CAD build for the part. Positions are in the model's coordinates, mm. Face numbers are marked on the shaded views. Coordinates: 2 decimals unless noted, no trailing zeros. Write each loop counter-clockwise with the first axis right and the second up, starting at its lowest first coordinate (ties: lowest second). Pieces come first, ordered by that corner, then holes.
```python
from build123d import *

# Parameters (mm, degrees)
F0_R          = 8.875
F1_DEPTH      = 5
F1_DEPTH_BACK = 5
F2_DEPTH      = 4
F2_DEPTH_BACK = 4
F3_SIZE       = 1


# Not quite as in the source:
# - a feature names something its author has since deleted; it is built from what else it names


with BuildPart() as f1:
    # F0 (on Front) → F1 (new body, two sides)
    with BuildSketch(Plane.XZ) as f1_sk:
        with BuildLine():
            ThreePointArc((-5, 9.0906889178), (-5.2804178338, -8.9307229551), (10.375, 0))
            ThreePointArc((10.375, 0), (8.9307229551, 5.2804178338), (5, 9.0906889178))
            Line((5, 9.0906889178), (5, 8.9453239366))
            Line((5, 8.9453239366), (-5, 8.9453239366))
            Line((-5, 8.9453239366), (-5, 9.0906889178))
        make_face()
        Circle(F0_R, mode=Mode.SUBTRACT)
        with BuildLine():
            Line((5, 8.9453239366), (5, 9.0906889178))
            ThreePointArc((5, 9.0906889178), (0, 10.375), (-5, 9.0906889178))
            Line((-5, 9.0906889178), (-5, 8.9453239366))
            Line((-5, 8.9453239366), (5, 8.9453239366))
        make_face()
    extrude(amount=F1_DEPTH)
    extrude(f1_sk.sketch, amount=-F1_DEPTH_BACK)

    # F0 (on Front) → F2 (join, two sides)
    with BuildSketch(Plane.XZ) as f2_sk:
        with BuildLine():
            ThreePointArc((-5, 9.0906889178), (0, 10.375), (5, 9.0906889178))
            Line((5, 9.0906889178), (5, 13.9453239366))
            Line((5, 13.9453239366), (-5, 13.9453239366))
            Line((-5, 13.9453239366), (-5, 9.0906889178))
        make_face()
    extrude(amount=F2_DEPTH)
    extrude(f2_sk.sketch, amount=-F2_DEPTH_BACK)

    # F3
    f3_edges = [f1.edges().sort_by_distance(p)[0] for p in [
        (-8.875, 5, 0),
        (-8.875, -5, 0),
    ]]
    chamfer(f3_edges, length=F3_SIZE)


solid = f1.part
```
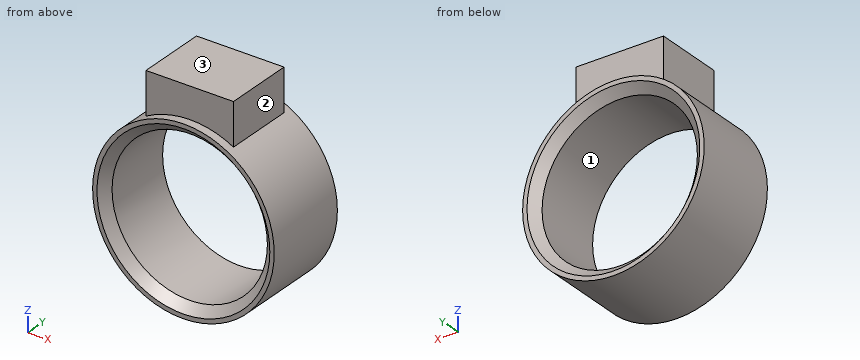
Item 1: Two-plate mould, pull along X, no slides. Class the marked faces 1, 2 and 3: +X half, -X half, draft (parallel to the pull), parting line (faces both ways), or undercut.
Item 2: Wall check: line 1 along Z through (x, y) = (0, 0.5) (3 decimals); line 2 along Z through (x, y) = (-4, -3.25); line 3 along X through (y, z) = (-3.5, -4.75). Give the ranges that are in metal, low to high.
Item 3: Flat gauge pins, fed straight in: pin 1 Ø3 at (x, y) = (4.5, 0) entering from -Z; pin 2 Ø2.5 at (x, z) = (2.5, 12) entering from +Y; pin 3 Ø1.5 at (y, z) = (1, 7.5) entering from -X. Where does each tip first touch, or does it go through?
Item 4: Saw through at B-B, the plane z = 0. Write the cut outline in (x, y) (3 decimals), and give its area (3 significant figures).
Item 5: Saw through at C-C, the plane y = -2.25. Write the cut outline in (x, z) (3 decimals), and give its area (3 significant figures).
Item 6: Saw through at A-A, the plane x = 0. Write the cut outline in (y, z) (3 decimals), and give its area (3 significant figures).
Working result:
1. face 1: undercut
1. face 2: +X half
1. face 3: draft
2. line 1: z = -10.375 to -8.875, 8.875 to 13.945
2. line 2: z = -9.57 to -7.92, 7.92 to 13.95
2. line 3: x = -9.22 to -7.5, 7.5 to 9.22
3. pin 1: stops at z = -9.93
3. pin 2: stops at y = 4
3. pin 3: stops at x = -7.88
4. outline: (-10.375, -5) - (-9.875, -5) - (-8.875, -4) - (-8.875, 4) - (-9.875, 5) - (-10.375, 5) - close; (8.875, -4) - (9.875, -5) - (10.375, -5) - (10.375, 5) - (9.875, 5) - (8.875, 4) - close
4. area: 28.0 mm2
5. outline: (-5, 9.091) arc R10.375 ccw (long way) to (5, 9.091) - (5, 13.945) - (-5, 13.945) - close; hole circle Ø17.75 at (0, 0)
5. area: 131 mm2
6. outline: (-5, -10.375) - (5, -10.375) - (5, -9.875) - (4, -8.875) - (-4, -8.875) - (-5, -9.875) - close; (-5, 9.875) - (-4, 8.875) - (4, 8.875) - (5, 9.875) - (5, 10.375) - (4, 10.375) - (4, 13.945) - (-4, 13.945) - (-4, 10.375) - (-5, 10.375) - close
6. area: 56.6 mm2
